Verification items for the finished model (mm, model axes). A direction names the side the tool comes from. Give positions to 0.01 mm unless a question says otherwise; leave off trailing zeros. Loops run counter-clockwise (first coordinate to the right, second up) from the corner with the lowest first, then second, coordinate; pieces in that order, holes last. Notation, with made-up numbers: M -11,-0.75 L 9,-0.75 A24 ccw 9,29.25 Z; hole C -20.5,61 d11. An arc over 180 degrees is marked long. Use CSV: the item, a comma, the result in double quotes.
from build123d import *

# Parameters (mm, degrees)
SKETCH007_R  = 1.7
PAD007_DEPTH = 13.5


with BuildPart() as obj1:
    # Sketch007 → Pad007 (new body)
    with BuildSketch(Plane(origin=(0, 19.25, 0), x_dir=(-1, 0, 0), z_dir=(0, 1, 0))):
        with BuildLine():
            ThreePointArc((59, 33), (55, 29), (59, 25))
            Line((59, 25), (84.428048, 25))
            Line((84.428048, 25), (98.820237, 15.646102))
            ThreePointArc((98.820237, 15.646102), (104.353886, 16.820218), (103.1798, 22.353874))
            Line((86.799351, 33), (103.1798, 22.353874))
            Line((59, 33), (86.799351, 33))
        make_face()
        with Locations((59, 29)):
            Circle(SKETCH007_R, mode=Mode.SUBTRACT)
        with Locations((101, 19)):
            Circle(SKETCH007_R, mode=Mode.SUBTRACT)
    extrude(amount=PAD007_DEPTH)


with BuildPart() as part_mirroring014:
    # Part__Mirroring014: instance of obj1
    add(obj1.part.mirror(Plane(origin=(0, 0, 0), x_dir=(0, -1, 0), z_dir=(1, 0, 0))))


with BuildPart() as part_mirroring022:
    # Part__Mirroring022: instance of Part__Mirroring014
    add(part_mirroring014.part.mirror(Plane(origin=(67.968658, 4e-06, 24.002777), x_dir=(1, 0, 0), z_dir=(0, 1, 0))))


solid = part_mirroring022.part
(1) Section check B-B on y = -29.5. Record the cut outline in (x, z).
Calculated:
outline,"M 59,25 L 84.43,25 L 98.82,15.65 A4 ccw 103.18,22.35 L 86.8,33 L 59,33 A4 ccw Z; hole C 59,29 d3.4; hole C 101,19 d3.4"
(2) Mould release check, pull along X, two halves, no side actions. Record for faces 3 (the cylindrical face through (99.3, -25.91, 19.07)), 4 (the cylindrical face through (57.3, -25.91, 29.07)), 5 (the flat face through (80, -19.25, 28)), 6 (the flat face through (91.52, -25.91, 20.39)): released by +X, released by -X, zero draft, split by the parting line, or undercut.
Calculated:
face 3,"undercut"
face 4,"undercut"
face 5,"zero draft"
face 6,"released by -X"
(3) Section check D-D on x = 77. Record the cut outline in (y, z), plus the area to 3 significant figures.
Calculated:
outline,"M -32.75,25 L -19.25,25 L -19.25,33 L -32.75,33 Z"
area,"108 mm²"
(4) Section check C-C on x = 101. Record the cut outline in (y, z), plus the area to 3 significant figures.
Calculated:
outline,"M -32.75,15 L -19.25,15 L -19.25,17.3 L -32.75,17.3 Z; M -32.75,20.7 L -19.25,20.7 L -19.25,23.77 L -32.75,23.77 Z"
area,"72.5 mm²"
(5) Tool access check on faces 1 (the cylindrical face through (55, -26, 29)), 2 (the flat face through (72, -26, 25)). Record the directions out of +Z, -Z, +X, -X, +Y, -Y that give a thin tool (end or side, any length) a straight path to the whole face; none if there is none.
Calculated:
face 1,"-X, +Y, -Y"
face 2,"-Z, -X, +Y, -Y"
(6) Depth check by flat-ended pin: pin 1 Ø6 at (x, y) = (84, -21) entering from -Z; pin 2 Ø1.5 at (x, y) = (90.5, -26) entering from +Z; pin 3 Ø5 at (x, y) = (67.5, -31.5) entering from -Z. Enter the tip coordinate at first touch or a pass-through.
Calculated:
pin 1,"stops at z = 23.33"
pin 2,"stops at z = 31.08"
pin 3,"stops at z = 25"
(7) Scan lines: L1, parallel to Z at x = 59, y = -21.75; L2, parallel to Z at x = 79.5, y = -27.25; L3, parallel to Z at x = 59.5, y = -28.25. Record each from-to range of solid material in increasing order. Write a range as from..to.
Calculated:
L1,"z = 25..27.3, 30.7..33"
L2,"z = 25..33"
L3,"z = 25..27.38, 30.62..33"
(8) Section check A-A on z = 19. Record the cut outline in (x, y).
Calculated:
outline,"M 93.66,-32.75 L 99.3,-32.75 L 99.3,-19.25 L 93.66,-19.25 Z; M 102.7,-32.75 L 105,-32.75 L 105,-19.25 L 102.7,-19.25 Z"
